```python
from build123d import *

# Parameters (mm, degrees)
F0_R     = 9.525
F1_DEPTH = 38.1
F0_R_2   = 6.35
F2_DEPTH = 12.7


# Not quite as in the source:
# - a feature of the source that left no trace in its solid (it failed there, or was rolled back) is left out


with BuildPart() as f1:
    # F0 (on Top) → F1 (new body)
    with BuildSketch(Plane.XY):
        with BuildLine():
            ThreePointArc((1.9538461538, -25.3247405753), (18.6385043969, -17.2559020004), (25.4, 0))
            ThreePointArc((25.4, 0), (18.6385043969, 17.2559020004), (1.9538461538, 25.3247405753))
            ThreePointArc((1.9538461538, 25.3247405753), (-25.4, 0), (1.9538461538, -25.3247405753))
        make_face()
        Circle(F0_R, mode=Mode.SUBTRACT)
    extrude(amount=F1_DEPTH)

    # F0 (on Top) → F2 (join)
    with BuildSketch(Plane.XY):
        with BuildLine():
            ThreePointArc((1.9538461538, -25.3247405753), (18.6385043969, -17.2559020004), (25.4, 0))
            ThreePointArc((25.4, 0), (18.6385043969, 17.2559020004), (1.9538461538, 25.3247405753))
            ThreePointArc((1.9538461538, 25.3247405753), (-25.4, 0), (1.9538461538, -25.3247405753))
        make_face()
        Circle(F0_R, mode=Mode.SUBTRACT)
        with BuildLine():
            ThreePointArc((1.9538461538, 25.3247405753), (18.6385043969, 17.2559020004), (25.4, 0))
            ThreePointArc((25.4, 0), (18.6385043969, -17.2559020004), (1.9538461538, -25.3247405753))
            Line((1.9538461538, -25.3247405753), (84.0153846154, -18.9935554315))
            ThreePointArc((84.0153846154, -18.9935554315), (63.5, 0), (84.0153846154, 18.9935554315))
            Line((84.0153846154, 18.9935554315), (1.9538461538, 25.3247405753))
        make_face()
        with BuildLine():
            ThreePointArc((101.6, 0), (96.5288782977, 12.9419265003), (84.0153846154, 18.9935554315))
            ThreePointArc((84.0153846154, 18.9935554315), (63.5, 0), (84.0153846154, -18.9935554315))
            ThreePointArc((84.0153846154, -18.9935554315), (96.5288782977, -12.9419265003), (101.6, 0))
        make_face()
        with Locations((82.55, 0)):
            Circle(F0_R_2, mode=Mode.SUBTRACT)
    extrude(amount=F2_DEPTH)


solid = f1.part
```
The model under review builds one solid part; all positions refer to its coordinate system, in mm. Round coordinates to 2 decimals unless told otherwise and drop trailing zeros. Loops run counter-clockwise (first coordinate to the right, second up) from the corner with the lowest first, then second, coordinate; pieces in that order, holes last. Notation, with made-up numbers: (76.25, 57) -> (111.25, 57) arc R21 cw to (111.25, 72) -> close; hole circle Ø5 at (-11.75, 16.5). An arc over 180 degrees is marked (long way). Answer as a JSON object with one key per item and string values. Group by question number.
1) We need section C-C on x = 19.5. Write out the cut boundary in (y, z).
2) We need section D-D on z = 33.5. Write out the cut boundary in (x, y) (3 decimals), then the cut area to 3 significant figures.
3) For line 1 (Y direction, x = 0, z = 9) (3 decimals); line 2 (X direction, y = -1, z = 2); line 3 (Z direction, x = 19.5, y = -22), list the stretches that pass through material, from the lowest coordinate up. Write a range as [from, to].
4) We need section B-B on x = 0. Write out the cut boundary in (y, z) (3 decimals), then the cut area to 3 significant figures.
5) For pin 1 Ø8 at (y, z) = (14.5, 26.5) entering from -X; pin 2 Ø8 at (x, z) = (7, 9) entering from -Y; pin 3 Ø12 at (x, z) = (59, 21.5) entering from -Y; pin 4 Ø10 at (y, z) = (12, 20.5) entering from -X, all flat-tipped, find the tip position at first contact; note any pin that passes through.
6) We need section A-A on z = 6.5. Write out the cut boundary in (x, y) (3 decimals), then the cut area to 3 significant figures.
7) Mouldability with a two-part tool opening along Y and no side actions: class faces 1 (the face through (43.559, 22.115, 6.261)), 2 (the face through (37, 0, 0)), 3 (the face through (76.206, 0.279, 6.261)) as released by +Y, released by -Y, zero draft, split by the parting line, or undercut.
Result set:
{
 "1": {"outline": "(-23.97, 0) -> (23.97, 0) -> (23.97, 12.7) -> (16.28, 12.7) -> (16.28, 38.1) -> (-16.28, 38.1) -> (-16.28, 12.7) -> (-23.97, 12.7) -> close"},
 "2": {"outline": "circle Ø50.8 at (0, 0); hole circle Ø19.05 at (0, 0)", "area": "1,740 mm²"},
 "3": {"line 1": "[-25.4, -9.525], [9.525, 25.4]", "line 2": "[-25.38, -9.47], [9.47, 76.28], [88.82, 101.57]", "line 3": "[0, 12.7]"},
 "4": {"outline": "(-25.4, 0) -> (-9.525, 0) -> (-9.525, 38.1) -> (-25.4, 38.1) -> close; (9.525, 0) -> (25.4, 0) -> (25.4, 38.1) -> (9.525, 38.1) -> close", "area": "1,210 mm²"},
 "5": {"pin 1": "x = -23.13", "pin 2": "y = -25.24", "pin 3": "through", "pin 4": "x = -24.42"},
 "6": {"outline": "(1.954, -25.325) -> (84.015, -18.994) arc R19.05 ccw to (84.015, 18.994) -> (1.954, 25.325) arc R25.4 ccw (long way) to start; hole circle Ø19.05 at (0, 0); hole circle Ø12.7 at (82.55, 0)", "area": "4,850 mm²"},
 "7": {"face 1": "released by +Y", "face 2": "zero draft", "face 3": "undercut"}
}
